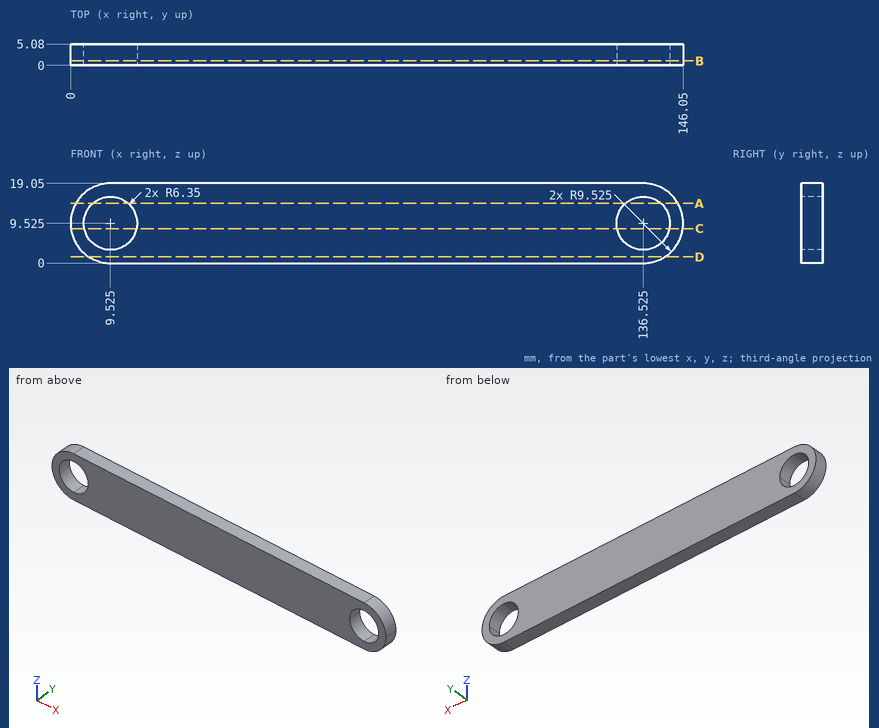
Can you work these out from the drawing? Everything is in mm from the part's minimum corner. Coordinates: 2 decimals unless noted, no trailing zeros. Write each loop counter-clockwise with the first axis right and the second up, starting at its lowest first coordinate (ties: lowest second). Pieces come first, ordered by that corner, then holes. Notation, with made-up numbers: (16, -20) -> (70, -20) arc R20 cw to (70, 4) -> close; hole circle Ø8 at (-20.5, 88.25). An arc over 180 degrees is marked (long way). Write each question's results on one line, items separated by ' | '. Start each with the question number.
Q1. Imagine slicing it at C-C (z = 8.25). Write out the boundary of the cut face in (x, y), then the cut area to 3 significant figures.
Q2. I'm going to push a flat-ended pin straight in: pin 1 (1 mm diameter, centred on y = 1.5, z = 3, fed in from +X). Where does the tip first touch, or does it pass through?
Q3. Imagine slicing it at B-B (y = 1.05). Write out the boundary of the cut face in (x, z) (3 decimals).
Q4. Imagine slicing it at D-D (z = 1.5). Write out the boundary of the cut face in (x, y).
Q5. If I drill on probe 1 along X at (y, z) = (1.35, 9); probe 2 along X at (y, z) = (3.6, 13); probe 3 along Z at (x, y) = (139, 2.1), over which ranges is the centre line in solid material (lowest first)?
Q6. Imagine slicing it at A-A (z = 14.25). Write out the boundary of the cut face in (x, y), then the cut area to 3 significant figures.
Taken from the geometry:
1) outline: (0.09, 0) -> (3.3, 0) -> (3.3, 5.08) -> (0.09, 5.08) -> close; (15.75, 0) -> (130.3, 0) -> (130.3, 5.08) -> (15.75, 5.08) -> close; (142.75, 0) -> (145.96, 0) -> (145.96, 5.08) -> (142.75, 5.08) -> close | area: 615 mm^2
2) pin 1: stops at x = 143.9
3) outline: (9.525, 0) -> (136.525, 0) arc R9.525 ccw to (136.525, 19.05) -> (9.525, 19.05) arc R9.525 ccw to start; hole circle Ø12.7 at (9.525, 9.525); hole circle Ø12.7 at (136.525, 9.525)
4) outline: (4.39, 0) -> (141.66, 0) -> (141.66, 5.08) -> (4.39, 5.08) -> close
5) probe 1: x = 0.01 to 3.2, 15.85 to 130.2, 142.85 to 146.04 | probe 2: x = 0.66 to 4.21, 14.84 to 131.21, 141.84 to 145.39 | probe 3: z = 0.33 to 3.68, 15.37 to 18.72
6) outline: (1.25, 0) -> (5.28, 0) -> (5.28, 5.08) -> (1.25, 5.08) -> close; (13.77, 0) -> (132.28, 0) -> (132.28, 5.08) -> (13.77, 5.08) -> close; (140.77, 0) -> (144.8, 0) -> (144.8, 5.08) -> (140.77, 5.08) -> close | area: 643 mm^2
